```python
from build123d import *

# Parameters (mm, degrees)
BASPROSKE_W                  = 7
BASPROSKE_H                  = 7
TOOTHCUT_DEPTH               = 13.124355653
TEETHCUTS_COUNT              = 12
TEETHCUTS_ANGLE              = 330
HUBNEAONESKE_R               = 4
HUBNEARONE_DEPTH             = 4
BORSKE_R                     = 2
BORE_DEPTH                   = 12.0000508
ESQUISSE1_R                  = 2
BOSS_EXTRU_1_DEPTH           = 4
R_P_TITION_CIRCULAIRE1_COUNT = 2
R_P_TITION_CIRCULAIRE1_ANGLE = 90


with BuildPart() as part:
    # BasProSke → Base-Revolve (revolve)
    with BuildSketch(Plane(origin=(0, 0, 0), x_dir=(1, 0, 0), z_dir=(0, 1, 0)), mode=Mode.PRIVATE) as base_revolve_sk:
        with Locations((3.5, 3.5)):
            Rectangle(BASPROSKE_W, BASPROSKE_H)
    revolve(base_revolve_sk.sketch.rotate(Axis((-10, 0, 0), (1, 0, 0)), 180), axis=Axis((-10, 0, 0), (1, 0, 0)))

    # TooCutSke → ToothCut (cut, through all)
    with BuildSketch(Plane(origin=(0, 0, 0), x_dir=(0, 0, -1), z_dir=(1, 0, 0))):
        with BuildLine():
            ThreePointArc((0.562207301, 4.715604304), (0, 4.749), (-0.562207301, 4.715604304))
            ThreePointArc((-0.562207301, 4.715604304), (-0.837528627, 5.917009812), (-1.672850686, 6.823328788))
            ThreePointArc((-1.672850686, 6.823328788), (0, 7.0254), (1.672850686, 6.823328788))
            ThreePointArc((1.672850686, 6.823328788), (0.837528627, 5.917009812), (0.562207301, 4.715604304))
        make_face()
    toothcut = extrude(amount=TOOTHCUT_DEPTH, mode=Mode.SUBTRACT)

    # TeethCuts: ToothCut ×12 about axis
    teethcuts_axis = Axis((-10, 0, 0), (1, 0, 0))
    for i in range(1, TEETHCUTS_COUNT):
        add(toothcut.rotate(teethcuts_axis, i * TEETHCUTS_ANGLE / (TEETHCUTS_COUNT - 1)), mode=Mode.SUBTRACT)

    # HubNeaOneSke → HubNearOne (add)
    with BuildSketch(Plane.ZY):
        with Locations(Location((0, 0, 0), (0, 0, 180))):
            Circle(HUBNEAONESKE_R)
    extrude(amount=HUBNEARONE_DEPTH)

    # BorSke → Bore (cut, symmetric)
    with BuildSketch(Plane(origin=(0, 0, 0), x_dir=(0, 0, -1), z_dir=(1, 0, 0))):
        with Locations(Location((0, 0, 0), (0, 0, 180))):
            Circle(BORSKE_R)
    extrude(amount=BORE_DEPTH, both=True, mode=Mode.SUBTRACT)

    # Esquisse1 → Boss.-Extru.1 (add)
    with BuildSketch(Plane(origin=(7, 0, 0), x_dir=(0, 0, -1), z_dir=(1, 0, 0))):
        with Locations(Location((0, 0, 0), (0, 0, 180))):
            Circle(ESQUISSE1_R)
    extrude(amount=-BOSS_EXTRU_1_DEPTH)

    # Esquisse5 → Trou pour taraudage pour trou taraudé M2x0.41 (revolve, cut)
    with BuildSketch(Plane(origin=(-2, -3.943103852, 0.672258885), x_dir=(0, -0.1680647213420592, -0.9857759631073463), z_dir=(1, 0, 0))):
        Polygon((0, 0), (0, 5.480688495), (0.8, 5), (0.8, 0), align=None)
    trou_pour_taraudage_pour_trou_taraud_m2 = revolve(axis=Axis((-2, -10.202781218, 1.739469866), (0, 0.9857759631073462, -0.1680647213420592)), mode=Mode.SUBTRACT)

    # Répétition circulaire1: Trou pour taraudage pour trou taraudé M2x0.41 ×2 about axis
    r_p_tition_circulaire1_axis = Axis((12.0000508, 0, 0), (-1, 0, 0))
    for i in range(1, R_P_TITION_CIRCULAIRE1_COUNT):
        add(trou_pour_taraudage_pour_trou_taraud_m2.rotate(r_p_tition_circulaire1_axis, i * R_P_TITION_CIRCULAIRE1_ANGLE / (R_P_TITION_CIRCULAIRE1_COUNT - 1)), mode=Mode.SUBTRACT)


solid = part.part
```
The listing builds one solid part. Answer for the finished solid, in the listing's coordinates (mm). A direction names the side the tool comes from. Round coordinates to 2 decimals unless told otherwise and drop trailing zeros. Loops run counter-clockwise (first coordinate to the right, second up) from the corner with the lowest first, then second, coordinate; pieces in that order, holes last.
Q1. For a pull along Y with two mould halves and no side action, classify faces 3 (the face through (3.451, -4.687, -3.655)), 4 (the face through (-1.972, 3.905, 0.867)), 5 (the face through (3.45, -2.23, -5.51)) as released by +Y, released by -Y, zero draft, split by the parting line, or undercut.
Q2. Section A-A, the plane y = 6 is taken. Determine the outline of the cut face in (x, z).
Q3. Which of the six approach directions +Z, -Z, +X, -X, +Y, -Y give full straight-line access (tool end or side, diameter ignored) to faces 1 (the face through (3, 0, 0)), 2 (the face through (-2.24, -0.26, 3.02))?
Q4. Find the intervals of material crossed by line 1 (Y direction, x = 1, z = 6.25); line 2 (Y direction, x = -0.75, z = 0); line 3 (Y direction, x = -2.25, z = 0), in increasing order.
Q5. Section B-B, the plane x = -3 is taken. Determine the outline of the cut face in (y, z), then the cut area to 3 significant figures.
Completed:
1. face 3: released by -Y
1. face 4: split by the parting line
1. face 5: undercut
2. outline: (0, -2.21) - (7, -2.21) - (7, -0.88) - (0, -0.88) - close; (0, 0.88) - (7, 0.88) - (7, 2.21) - (0, 2.21) - close
3. face 1: -X
3. face 2: none
4. line 1: y = -2.16 to -1.05, 1.05 to 2.16
4. line 2: y = -4 to -2, 2 to 4
4. line 3: y = 2 to 4
5. outline: circle Ø8 at (0, 0); hole circle Ø4 at (0, 0)
5. area: 37.7 mm2
